Could you check a few things on this model? Use its own coordinates, in mm. A direction names the side the tool comes from. Round coordinates to 2 decimals unless told otherwise and drop trailing zeros. Loops run counter-clockwise (first coordinate to the right, second up) from the corner with the lowest first, then second, coordinate; pieces in that order, holes last.
from build123d import *

# Parameters (mm, degrees)
SKETCH1_W           = 330
SKETCH1_H           = 105
BOSS_EXTRUDE1_DEPTH = 230
SKETCH2_W           = 200
SKETCH2_H           = 230
BOSS_EXTRUDE2_DEPTH = 20
SKETCH5_R           = 9
BOSS_EXTRUDE4_DEPTH = 28
SKETCH5_5_R         = 15
BOSS_EXTRUDE5_DEPTH = 17
BOSS_EXTRUDE6_DEPTH = 36.5
MIRROR1_START       = 20.04628694
MIRROR1_OUTLINE_W   = 36.5
MIRROR1_OUTLINE_H   = 38.2
MIRROR1_DEPTH       = 38.2
MIRROR1_START_2     = 99.242246433
MIRROR1_2_OUTLINE_W = 36.5
MIRROR1_2_OUTLINE_H = 38.2
MIRROR1_2_DEPTH     = 38.2


# Read off the part's stored shape, not the designer's step: Mirror1
with BuildPart() as part:
    # Sketch1 → Boss-Extrude1 (new body)
    with BuildSketch(Plane.XY):
        Rectangle(SKETCH1_W, SKETCH1_H)
    extrude(amount=BOSS_EXTRUDE1_DEPTH)

    # Sketch2 → Boss-Extrude2 (add)
    with BuildSketch(Plane(origin=(0, 52.5, 0), x_dir=(1, 0, 0), z_dir=(0, 1, 0))):
        with Locations((40, -115)):
            Rectangle(SKETCH2_W, SKETCH2_H)
    extrude(amount=BOSS_EXTRUDE2_DEPTH)

    # Sketch5 → Boss-Extrude4 (add)
    with BuildSketch(Plane.XY.offset(230)):
        with Locations((115.5, 62.5)):
            Circle(SKETCH5_R)
        with Locations((-36, 62.5)):
            Circle(SKETCH5_R)
    extrude(amount=BOSS_EXTRUDE4_DEPTH)

    # Sketch5<5> → Boss-Extrude5 (add)
    with BuildSketch(Plane.XY.offset(230)):
        with Locations((-5, 0.5)):
            Circle(SKETCH5_5_R)
    extrude(amount=BOSS_EXTRUDE5_DEPTH)

    # Sketch6 → Boss-Extrude6 (add)
    with BuildSketch(Plane(origin=(165, 0, 0), x_dir=(0, 0, -1), z_dir=(1, 0, 0))):
        Polygon((-86.011479041, -3.638790093), (-59, -30.650269134), (-31.988520959, -3.638790093), (-59, 23.372688948), align=None)
        Polygon((-142.011479041, -3.638790093), (-115, -30.650269134), (-87.988520959, -3.638790093), (-115, 23.372688948), align=None)
        Polygon((-198.011479041, -3.638790093), (-171, -30.650269134), (-143.988520959, -3.638790093), (-171, 23.372688948), align=None)
    extrude(amount=BOSS_EXTRUDE6_DEPTH)

    # Mirror1 outline → Mirror1 (add)
    with BuildSketch(Plane(origin=(0, 0, 0), x_dir=(1, 0, 0), z_dir=(0, 0.707106781186546, 0.707106781186549)).offset(MIRROR1_START)):
        with Locations((-183.25, -44.29231324)):
            Rectangle(MIRROR1_OUTLINE_W, MIRROR1_OUTLINE_H)
    extrude(amount=MIRROR1_DEPTH)

    # Mirror1 2 outline → Mirror1 2 (add)
    with BuildSketch(Plane(origin=(0, 0, 0), x_dir=(1, 0, 0), z_dir=(0, 0.707106781186546, 0.707106781186549)).offset(MIRROR1_START_2)):
        with Locations((-183.25, -123.488272733)):
            Rectangle(MIRROR1_2_OUTLINE_W, MIRROR1_2_OUTLINE_H)
    extrude(amount=MIRROR1_2_DEPTH)


solid = part.part
Item 1: If we section it at D-D, the plane x = -5: Please give me the cut outline in (y, z), then the cut area to 3 significant figures.
Results list:
outline: (-52.5, 0) - (72.5, 0) - (72.5, 230) - (15.5, 230) - (15.5, 247) - (-14.5, 247) - (-14.5, 230) - (-52.5, 230) - close
area: 29,300 mm2
Item 2: For faces 1 (the flat face through (-183.505, 10.056, 184.317)), 2 (the flat face through (182.99, -17.33, 45.68)), 3 (the flat face through (-183.51, -16.96, 157.31)), 4 (the flat face through (182.994, 10.056, 72.317)), 5 (the cylindrical face through (8.856, -5.245, 238.381)), which set-ups out of +Z, -Z, +X, -X, +Y, -Y let a thin tool reach every point of the face, with its end or its side?
Results list:
face 1: +Z, -X, +Y
face 2: -Z, +X, -Y
face 3: -X, -Y
face 4: +X, +Y
face 5: +Z
Item 3: If I drill on line 1 along Z through (x, y) = (167, -21.5); line 2 along Y through (x, z) = (-103, 149.5); line 3 along X through (y, z) = (-35.5, 167), over which ranges is the centre line in solid material (lowest first)?
Results list:
line 1: z = 49.85 to 68.15, 105.85 to 124.15, 161.85 to 180.15
line 2: y = -52.5 to 52.5
line 3: x = -165 to 165
Item 4: If we section it at C-C, the plane z = 92: Please give me the cut outline in (x, y), then the cut area to 3 significant figures.
Results list:
outline: (-165, -52.5) - (165, -52.5) - (165, -7.65) - (201.5, -7.65) - (201.5, 0.37) - (165, 0.37) - (165, 52.5) - (140, 52.5) - (140, 72.5) - (-60, 72.5) - (-60, 52.5) - (-165, 52.5) - close
area: 38,900 mm2
Item 5: If we section it at A-A, the plane x = 115.5: Please give me the cut outline in (y, z), then the cut area to 3 significant figures.
Results list:
outline: (-52.5, 0) - (72.5, 0) - (72.5, 230) - (71.5, 230) - (71.5, 258) - (53.5, 258) - (53.5, 230) - (-52.5, 230) - close
area: 29,300 mm2
Item 6: Will these pins go through, and if not, where does the flat tip stop? pin 1 (12 mm diameter, centred on x = -23.5, y = -3, fed in from +Z); pin 2 (1 mm diameter, centred on y = -34, z = 168, fed in from -X); pin 3 (4 mm diameter, centred on x = -127, z = 41.5, fed in from +Y).
Results list:
pin 1: stops at z = 247
pin 2: stops at x = -165
pin 3: stops at y = 52.5
Item 7: If we section it at B-B, the plane y = 62.5: Please give me the cut outline in (x, z).
Results list:
outline: (-60, 0) - (140, 0) - (140, 230) - (124.5, 230) - (124.5, 258) - (106.5, 258) - (106.5, 230) - (-27, 230) - (-27, 258) - (-45, 258) - (-45, 230) - (-60, 230) - close
